```python
from build123d import *

# Parameters (mm, degrees)
ESBO_O1_W                = 80
ESBO_O1_H                = 120
RESSALTO_EXTRUS_O1_DEPTH = 15
FILETE1_R                = 15
ESBO_O2_R                = 7.5
CORTE_EXTRUS_O1_DEPTH    = 146


with BuildPart() as part:
    # Esboço1 → Ressalto-extrusão1 (new body)
    with BuildSketch(Plane(origin=(0, 0, 0), x_dir=(1, 0, 0), z_dir=(0, 1, 0))):
        with Locations((40, 60)):
            Rectangle(ESBO_O1_W, ESBO_O1_H)
    extrude(amount=RESSALTO_EXTRUS_O1_DEPTH)

    # Filete1
    filete1_edges = [part.edges().sort_by_distance(p)[0] for p in [
        (0, 7.5, -120),
        (80, 7.5, -120),
        (80, 7.5, 0),
        (0, 7.5, 0),
    ]]
    fillet(filete1_edges, radius=FILETE1_R)

    # Esboço2 → Corte-extrusão1 (cut, through all)
    with BuildSketch(Plane(origin=(0, 15, 0), x_dir=(1, 0, 0), z_dir=(0, 1, 0))):
        with Locations(Location((15, 105, 0), (0, 0, 270))):
            Circle(ESBO_O2_R)
        with Locations(Location((65, 105, 0), (0, 0, 270))):
            Circle(ESBO_O2_R)
        with Locations(Location((65, 60, 0), (0, 0, 270))):
            Circle(ESBO_O2_R)
        with Locations(Location((65, 15, 0), (0, 0, 270))):
            Circle(ESBO_O2_R)
        with Locations(Location((15, 60, 0), (0, 0, 270))):
            Circle(ESBO_O2_R)
        with Locations(Location((15, 15, 0), (0, 0, 270))):
            Circle(ESBO_O2_R)
    extrude(amount=-CORTE_EXTRUS_O1_DEPTH, mode=Mode.SUBTRACT)


solid = part.part
```
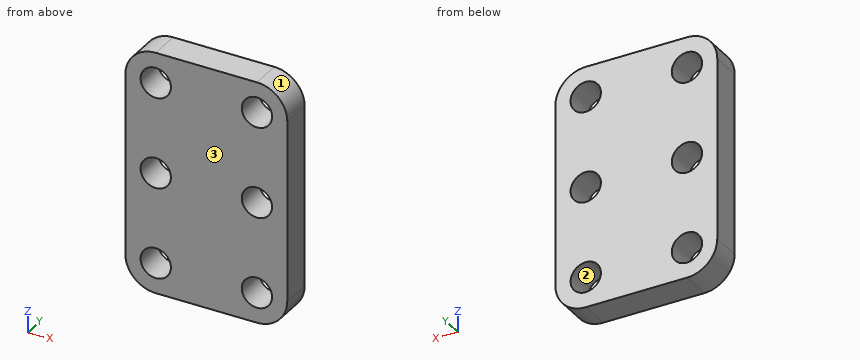
Geometry check sheet. Reference: the model listing, model coordinates, mm. Face numbers are marked on the shaded views. Coordinates: 2 decimals unless noted, no trailing zeros. Order: outer loops, then holes, each group sorted by start corner. A loop starts at its lowest first (then second) coordinate and runs counter-clockwise, first axis right, second up.
Q1. Draft check along X on the marked faces 1, 2 and 3. Enter one of: released by +X, released by -X, zero draft, split by the parting line, or undercut.
Reply:
face 1: released by +X
face 2: undercut
face 3: zero draft
Q2. Sectioned sample at A-A on z = -60. Record the cut outline in (x, y).
Reply:
outline: (0, 0) - (7.5, 0) - (7.5, 15) - (0, 15) - close; (22.5, 0) - (57.5, 0) - (57.5, 15) - (22.5, 15) - close; (72.5, 0) - (80, 0) - (80, 15) - (72.5, 15) - close
Q3. Sectioned sample at C-C on y = 13.75. Record the cut outline in (x, z), and give its area (3 significant figures).
Reply:
outline: (0, -105) arc R15 ccw to (15, -120) - (65, -120) arc R15 ccw to (80, -105) - (80, -15) arc R15 ccw to (65, 0) - (15, 0) arc R15 ccw to (0, -15) - close; hole circle Ø15 at (15, -105); hole circle Ø15 at (15, -60); hole circle Ø15 at (15, -15); hole circle Ø15 at (65, -105); hole circle Ø15 at (65, -60); hole circle Ø15 at (65, -15)
area: 8,350 mm2
Q4. Sectioned sample at B-B on x = 67.5. Record the cut outline in (y, z), and give its area (3 significant figures).
Reply:
outline: (0, -119.79) - (15, -119.79) - (15, -112.07) - (0, -112.07) - close; (0, -97.93) - (15, -97.93) - (15, -67.07) - (0, -67.07) - close; (0, -52.93) - (15, -52.93) - (15, -22.07) - (0, -22.07) - close; (0, -7.93) - (15, -7.93) - (15, -0.21) - (0, -0.21) - close
area: 1,160 mm2
Q5. Sectioned sample at D-D on x = 10.5. Record the cut outline in (y, z), and give its area (3 significant figures).
Reply:
outline: (0, -119.31) - (15, -119.31) - (15, -111) - (0, -111) - close; (0, -99) - (15, -99) - (15, -66) - (0, -66) - close; (0, -54) - (15, -54) - (15, -21) - (0, -21) - close; (0, -9) - (15, -9) - (15, -0.69) - (0, -0.69) - close
area: 1,240 mm2
Q6. Thickness scan on probe 1 along X at (y, z) = (10.25, -60); probe 2 along Z at (x, y) = (17, 5); probe 3 along X at (y, z) = (1.75, -64.5). Record the ranges inside material, lowest first.
Reply:
probe 1: x = 0 to 7.5, 22.5 to 57.5, 72.5 to 80
probe 2: z = -120 to -112.23, -97.77 to -67.23, -52.77 to -22.23, -7.77 to 0
probe 3: x = 0 to 9, 21 to 59, 71 to 80
